Study the drawing (mm; zero at the part's minimum x, y, z) and answer. Round coordinates to 2 decimals unless told otherwise and drop trailing zeros. Loops run counter-clockwise (first coordinate to the right, second up) from the corner with the lowest first, then second, coordinate; pieces in that order, holes last. Notation, with made-up numbers: M 15,57 L 64,57 A33 ccw 64,92 Z; hole C 9.25,-34 d8. An arc over 180 degrees is marked long. Write each question's results on one line, items separated by ' | '.
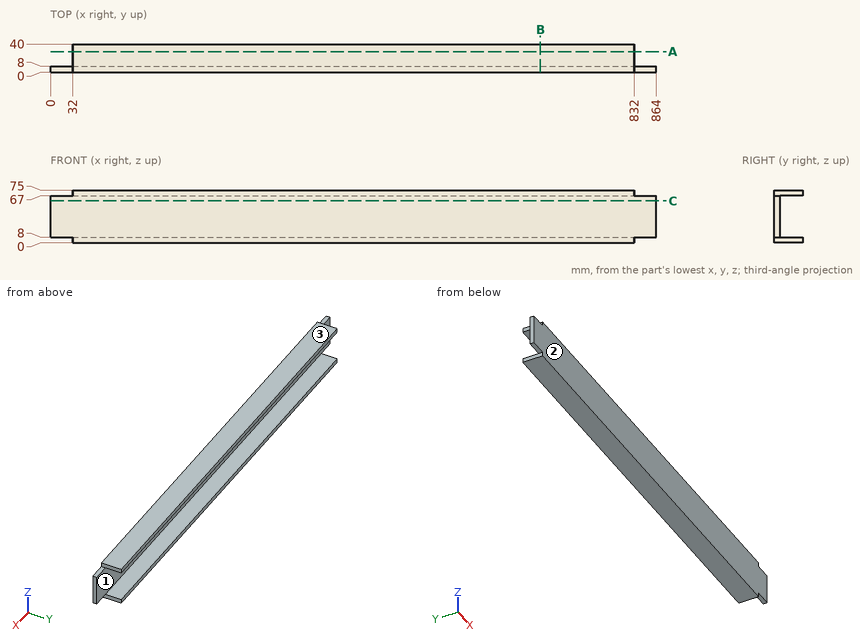
Item 1: The part is cut by section A-A (y = 29). Determine the outline of the cut face in (x, z).
Outcome:
outline: M 32,0 L 832,0 L 832,8 L 32,8 Z; M 32,67 L 832,67 L 832,75 L 32,75 Z
Item 2: Straight lines are drawn through the part: line 1 (Z direction, x = 39, y = 13.5); line 2 (Y direction, x = 414, z = 54); line 3 (X direction, y = 3.5, z = 67.5). For each, find the intervals that lie inside material, in ascending order.
Outcome:
line 1: z = 0 to 8, 67 to 75 | line 2: y = 0 to 8 | line 3: x = 32 to 832
Item 3: The part is cut by section C-C (z = 59.5). Determine the outline of the cut face in (x, y).
Outcome:
outline: M 0,0 L 864,0 L 864,8 L 0,8 Z
Item 4: The mould has two halves that part along Z. Classify the marked faces 1, 2 and 3: pulls with the +Z half, pulls with the -Z half, needs draft (parallel to the pull), parting line crosses it, or undercut.
Outcome:
face 1: undercut | face 2: needs draft | face 3: pulls with the +Z half
Item 5: Flat-ended cylindrical pins translate along their axes: pin 1 (6.5 mm diameter, centred on y = 21, z = 3.5, fed in from -X); pin 2 (4 mm diameter, centred on x = 854.5, y = 2.5, fed in from -Z); pin 3 (9 mm diameter, centred on x = 18.5, y = 4.5, fed in from +Z). Find the tip coordinate at first contact, or state that the pin passes through.
Outcome:
pin 1: stops at x = 32 | pin 2: stops at z = 8 | pin 3: stops at z = 67
Item 6: The part is cut by section B-B (x = 698.5). Determine the outline of the cut face in (y, z).
Outcome:
outline: M 0,0 L 40,0 L 40,8 L 8,8 L 8,67 L 40,67 L 40,75 L 0,75 Z
